The figure shows three views and two pictorial views of one solid part (mm, origin at its lowest corner). Answer the questions. A direction names the side the tool comes from. Give positions to 0.01 mm unless a question says otherwise; leave off trailing zeros. Write each loop counter-clockwise with the first axis right and the second up, starting at its lowest first coordinate (ties: lowest second). Pieces come first, ordered by that corner, then holes. Notation, with made-up numbers: (63.25, 16) -> (89.25, 16) arc R13 ccw to (89.25, 34) -> close; hole circle Ø5 at (26.5, 13). An arc over 180 degrees is marked (long way). Answer as CSV lines item,"result". Start each with the question number.
1. The part is cut by section C-C, the plane x = 40.5. Determine the outline of the cut face in (y, z).
2. Given pin 1 (5 mm diameter, centred on y = 17.5, z = 13.5, fed in from -X); pin 2 (4 mm diameter, centred on x = 16.5, z = 4.5, fed in from +Y); pin 3 (3 mm diameter, centred on x = 5, z = 5, fed in from +Y), each flat-ended and moving along its own axis, determine where each tip first touches the part or whether it passes through.
3. The part is cut by section A-A, the plane z = 10. Determine the outline of the cut face in (x, y), and give its area (4 significant figures).
4. A tool of negligible diameter and unlimited length cuts with its end or side. For the marked faces 1, 2, 3, 4 and 5, from which of +Z, -Z, +X, -X, +Y, -Y can it reach the whole face along a straight path? Write none if from no direction.
5. The part is cut by section D-D, the plane y = 33. Determine the outline of the cut face in (x, z).
6. The part is cut by section B-B, the plane y = 26. Determine the outline of the cut face in (x, z), and give its area (3 significant figures).
7. For a pull along X with two mould halves and no side action, classify the marked faces 6, 7 and 8 as pulls with the +X half, pulls with the -X half, needs draft (parallel to the pull), parting line crosses it, or undercut.
8. Find the intervals of material crossed by line 1 (X direction, y = 34, z = 15); line 2 (X direction, y = 1.8, z = 10); line 3 (X direction, y = 32, z = 2.5), in increasing order.
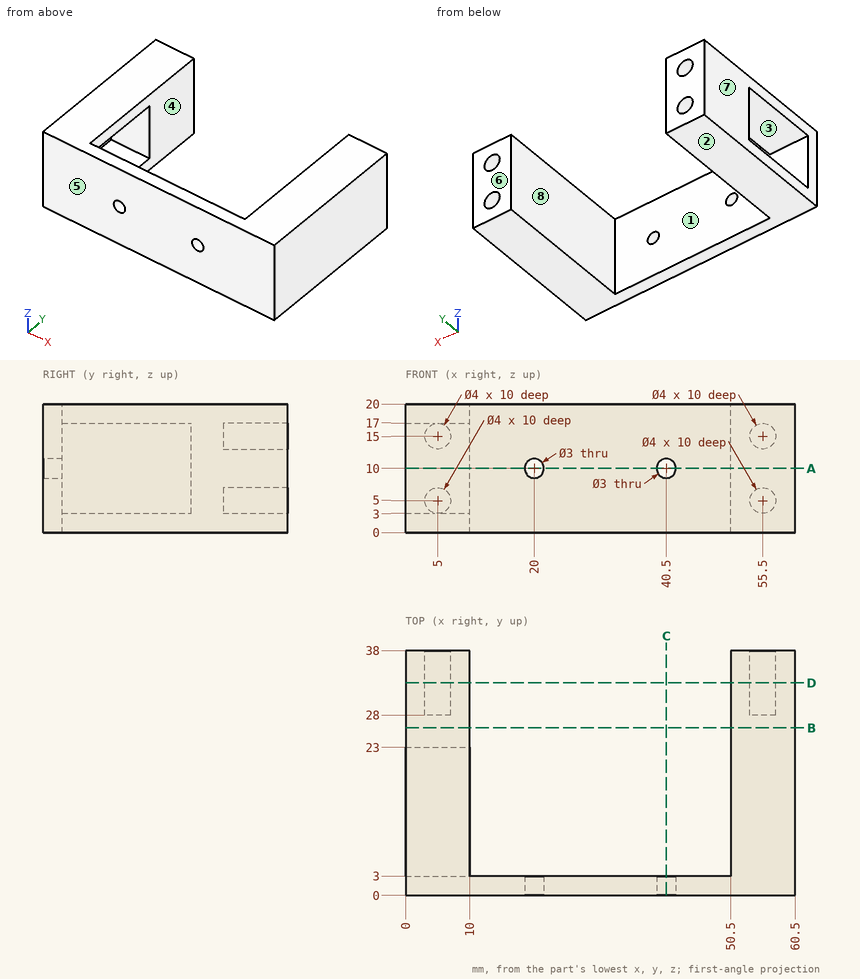
Results found:
1,outline,"(0, 0) -> (3, 0) -> (3, 8.5) -> (0, 8.5) -> close; (0, 11.5) -> (3, 11.5) -> (3, 20) -> (0, 20) -> close"
2,pin 1,"stops at x = 50.5"
2,pin 2,"stops at y = 3"
2,pin 3,"stops at y = 28"
3,outline,"(0, 0) -> (18.5, 0) -> (18.5, 3) -> (0, 3) -> close; (0, 23) -> (10, 23) -> (10, 38) -> (0, 38) -> close; (21.5, 0) -> (39, 0) -> (39, 3) -> (21.5, 3) -> close; (42, 0) -> (60.5, 0) -> (60.5, 38) -> (50.5, 38) -> (50.5, 3) -> (42, 3) -> close"
3,area,"663.5 mm²"
4,face 1,"none"
4,face 2,"-Z, +X, -X, +Y, -Y"
4,face 3,"-X"
4,face 4,"+Z, -Z, +Y"
4,face 5,"+Z, -Z, +X, -X, -Y"
5,outline,"(0, 0) -> (10, 0) -> (10, 20) -> (0, 20) -> close; (50.5, 0) -> (60.5, 0) -> (60.5, 20) -> (50.5, 20) -> close; hole circle Ø4 at (5, 5); hole circle Ø4 at (5, 15); hole circle Ø4 at (55.5, 5); hole circle Ø4 at (55.5, 15)"
6,outline,"(0, 0) -> (10, 0) -> (10, 20) -> (0, 20) -> close; (50.5, 0) -> (60.5, 0) -> (60.5, 20) -> (50.5, 20) -> close"
6,area,"400 mm²"
7,face 6,"needs draft"
7,face 7,"pulls with the -X half"
7,face 8,"undercut"
8,line 1,"x = 0 to 3, 7 to 10, 50.5 to 53.5, 57.5 to 60.5"
8,line 2,"x = 0 to 18.5, 21.5 to 39, 42 to 60.5"
8,line 3,"x = 0 to 10, 50.5 to 60.5"
